Part model, mm, in its own coordinate system. A direction names the side the tool comes from. Give positions to 0.01 mm unless a question says otherwise; leave off trailing zeros. Order: outer loops, then holes, each group sorted by start corner. A loop starts at its lowest first (then second) coordinate and runs counter-clockwise, first axis right, second up. Notation, with made-up numbers: M 12.5,-28.75 L 46.5,-28.75 A26 cw 46.5,-9.75 Z; hole C 20.5,-34 d7. An arc over 180 degrees is marked long. Answer as a JSON object with one key per item and string values.
Autodesk Inventor part; units mm, degrees
ref_plane "YZ Plane" through (0, 0, 0) normal (1, 0, 0) x (0, 1, 0)
ref_plane "XZ Plane" through (0, 0, 0) normal (0, 1, 0) x (-1, 0, 0)
ref_plane "XY Plane" through (0, 0, 0) normal (0, 0, 1) x (1, 0, 0)
sketch "Sketch1" plane through (0, 0, 0) normal (0, 1, 0) x (-1, 0, 0)
  circle A0 centre (0, 0) radius 27.5
  circle A1 centre (0, 0) radius 29
  dimension "d0" = 55
  dimension "d1" = 58
extrude "Extrusion1" add sketch "Sketch1" along normal blind 2.5 contours A0
extrude "Extrusion2" add sketch "Sketch1" along normal blind 20
sketch "Sketch3" plane through (0, 0, 0) normal (1, 0, 0) x (0, 1, 0)
  circle A0 centre (10, 0) radius 2.5
  line L0 (0, -29) -> (0, 29)
  point P0 (0, 0)
  dimension "d6" = 5
  dimension "d7" = 10
extrude "Extrusion3" cut sketch "Sketch3" along normal through all both and the other way through all
properties part number "Tapa_Tubo_PVC"
1. Pin check, flat tips, straight feed: P1, Ø8, axis at x = 8.5, y = 15.5, coming from the +Z side; P2, Ø1.5, axis at y = 8, z = 4.5, coming from the -X side; P3, Ø3, axis at x = -11.5, y = 4, coming from the -Z side. Stop position of each tip, or through.
Worked answers:
{"P1": "stops at z = 28.65", "P2": "stops at x = -28.76", "P3": "stops at z = -27.22"}
2. Probe line 1 along Z through (x, y) = (0, 10.5); line 2 along Z through (x, y) = (-11, 11). List the from-to ranges inside material, lowest first.
Worked answers:
{"line 1": "z = -29 to -27.5, 27.5 to 29", "line 2": "z = -26.83 to -25.2, 25.2 to 26.83"}
3. Cut at B-B on x = 0. Give the cut face in (y, z).
Worked answers:
{"outline": "M 0,-29 L 20,-29 L 20,-27.5 L 2.5,-27.5 L 2.5,27.5 L 20,27.5 L 20,29 L 0,29 Z"}
4. Which spindle directions (+Z, -Z, +X, -X, +Y, -Y) get a long thin tool onto all of the face, cutting with end or side? Do faces 1 (the cylindrical face through (-28.2, 7.5, 0.1)), 2 (the cylindrical face through (-25.403, 11.128, 10.533)). Say none if no direction does.
Worked answers:
{"face 1": "+X, -X", "face 2": "+Y"}
5. Two-plate mould, pull along Z, no slides. Class faces 3 (the flat face through (0, 2.5, 0)), 4 (the flat face through (0, 0, 0)), 5 (the cylindrical face through (-27.66, 9.86, -8.71)): +Z half, -Z half, draft (parallel to the pull), parting line (faces both ways), or undercut.
Worked answers:
{"face 3": "undercut", "face 4": "draft", "face 5": "parting line"}
6. Cut at D-D on y = 1.5. Give the cut face in (x, z), plus the area to 3 significant figures.
Worked answers:
{"outline": "C 0,0 d58", "area": "2,640 mm^2"}
7. Cut at A-A on z = 0. Give the cut face in (x, y).
Worked answers:
{"outline": "M -29,0 L 29,0 L 29,7.5 L 27.5,7.5 L 27.5,2.5 L -27.5,2.5 L -27.5,7.5 L -29,7.5 Z; M -29,12.5 L -27.5,12.5 L -27.5,20 L -29,20 Z; M 27.5,12.5 L 29,12.5 L 29,20 L 27.5,20 Z"}
